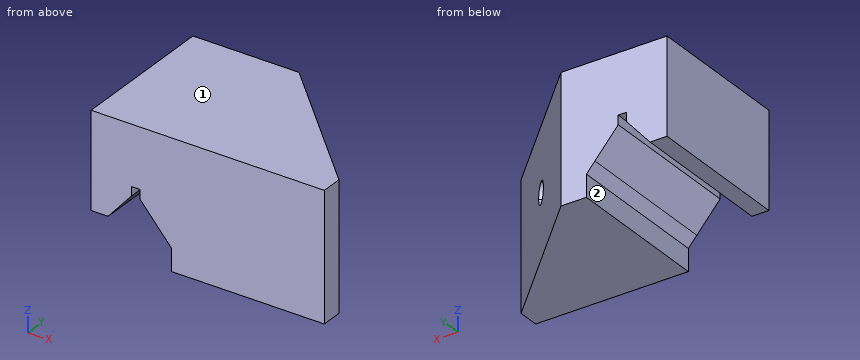
from build123d import *

# Parameters (mm, degrees)
F1_DEPTH = 44.45
F3_DEPTH = 38.1
F5_DEPTH = 12.7


with BuildPart() as f1:
    # F0 (on Front) → F1 (new body)
    with BuildSketch(Plane.XZ):
        Polygon((24.13, 6.594231), (24.13, 0), (69.85, 0), (69.85, 38.1), (0, 38.1), (0, 9.525), (5.08, 9.525), (12.065, 17.584615), (12.065, 19.05), (12.065, 20.32), (14.605, 20.32), (14.605, 19.05), (14.605, 17.584615), (21.59, 9.525), align=None)
    extrude(amount=F1_DEPTH)

    # F2 (on face) → F3 (cut)
    with BuildSketch(Plane.XY.offset(38.1)):
        Polygon((69.85, -38.1), (69.85, 0), (31.75, 0), align=None)
    extrude(amount=-F3_DEPTH, mode=Mode.SUBTRACT)

    # F4 (on face) → F5 (cut)
    with BuildSketch(Plane(origin=(15.875, 15.875, 0), x_dir=(-0.707107, 0.707107, 0), z_dir=(0.707107, 0.707107, 0))):
        with BuildLine():
            ThreePointArc((-49.391409, 22.225), (-51.636473, 21.295064), (-52.566409, 19.05))
            Line((-52.566409, 19.05), (-49.391409, 19.05))
            Line((-49.391409, 19.05), (-49.391409, 22.225))
        make_face()
        with BuildLine():
            Line((-49.391409, 19.05), (-52.566409, 19.05))
            ThreePointArc((-52.566409, 19.05), (-51.636473, 16.804936), (-49.391409, 15.875))
            Line((-49.391409, 15.875), (-49.391409, 19.05))
        make_face()
        with BuildLine():
            Line((-49.391409, 22.225), (-49.391409, 19.05))
            Line((-49.391409, 19.05), (-46.216409, 19.05))
            ThreePointArc((-46.216409, 19.05), (-47.146345, 21.295064), (-49.391409, 22.225))
        make_face()
        with BuildLine():
            Line((-46.216409, 19.05), (-49.391409, 19.05))
            Line((-49.391409, 19.05), (-49.391409, 15.875))
            ThreePointArc((-49.391409, 15.875), (-47.146345, 16.804936), (-46.216409, 19.05))
        make_face()
    extrude(amount=-F5_DEPTH, mode=Mode.SUBTRACT)


solid = f1.part
Verification items for the finished model (mm, model axes). Face numbers are marked on the shaded views. A direction names the side the tool comes from. Give positions to 0.01 mm unless a question says otherwise; leave off trailing zeros. Write each loop counter-clockwise with the first axis right and the second up, starting at its lowest first coordinate (ties: lowest second). Pieces come first, ordered by that corner, then holes. Notation, with made-up numbers: M 40,77.25 L 89,77.25 A17 cw 89,85.25 Z; hole C -18.75,-0.75 d3. An arc over 180 degrees is marked long. Put each result on its own line as item: value. Start each with the question number.
1. Section check D-D (y = -32.5). Record the cut outline in (x, z) (3 decimals), and give its area (3 significant figures).
2. Section check C-C (x = 34). Record the cut outline in (y, z), and give its area (3 significant figures).
3. Set-up check for the marked faces 1 and 2: record each of +Z, -Z, +X, -X, +Y, -Y from which the full face is reachable in a straight line by a thin tool's end or side.
4. Section check B-B (z = 31.5). Record the cut outline in (x, y), and give its area (3 significant figures).
5. Go/stop test with flat-tipped pins: pin 1 Ø12 at (y, z) = (-25, 24.5) entering from +X; pin 2 Ø7.5 at (y, z) = (-19, 3) entering from -X (3 decimals); pin 3 Ø1.5 at (x, y) = (2, -33) entering from -Z (3 decimals). Record where each tip stops, or that it passes through.
6. Scan lines: line 1 along X through (y, z) = (-27, 17); line 2 along X through (y, z) = (-41.5, 18) (3 decimals); line 3 along X through (y, z) = (-19, 10.5) (3 decimals). Record each from-to range of solid material in increasing order. Write a range as [from, to].
7. Section check A-A (y = -2.5). Record the cut outline in (x, z) (3 decimals).
Answer list:
1. outline: M 0,9.525 L 5.08,9.525 L 12.065,17.585 L 12.065,20.32 L 14.605,20.32 L 14.605,17.585 L 24.13,6.594 L 24.13,0 L 64.25,0 L 64.25,38.1 L 0,38.1 Z
1. area: 2,140 mm2
2. outline: M -44.45,0 L -2.25,0 L -2.25,38.1 L -44.45,38.1 Z
2. area: 1,610 mm2
3. face 1: +Z, +X, -X, +Y, -Y
3. face 2: -Z, -X, +Y, -Y
4. outline: M 0,-44.45 L 69.85,-44.45 L 69.85,-38.1 L 31.75,0 L 0,0 Z
4. area: 2,380 mm2
5. pin 1: x = 62.75
5. pin 2: x = 23.995
5. pin 3: z = 9.525
6. line 1: [0, 11.56], [15.11, 40.79], [46.28, 58.75]
6. line 2: [0, 12.065], [14.605, 69.85]
6. line 3: [0, 5.925], [20.745, 50.75]
7. outline: M 0,9.525 L 5.08,9.525 L 12.065,17.585 L 12.065,20.32 L 14.605,20.32 L 14.605,17.585 L 24.13,6.594 L 24.13,0 L 34.25,0 L 34.25,38.1 L 0,38.1 Z
